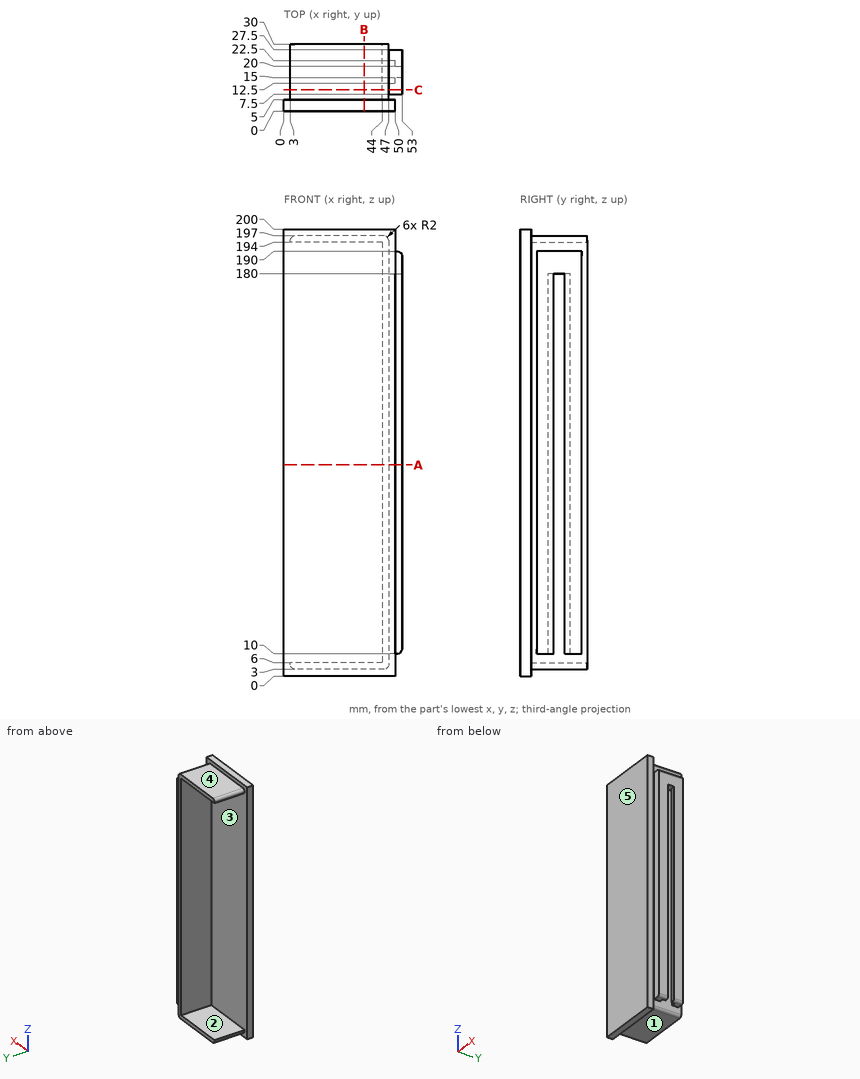
Here's the drawing with two shaded views (mm, measured from the low corner). I have some questions. A direction names the side the tool comes from. Give positions to 0.01 mm unless a question says otherwise; leave off trailing zeros. Write each loop counter-clockwise with the first axis right and the second up, starting at its lowest first coordinate (ties: lowest second). Pieces come first, ordered by that corner, then holes. Notation, with made-up numbers: (-30, 14.25) -> (0, 14.25) arc R25 cw to (0, 37.25) -> close; hole circle Ø5 at (89, -29). An arc over 180 degrees is marked (long way). Use one line per item in the form item = value.
1) Suppose I cut it at A-A (z = 94.5). Please give me the cut outline in (x, y).
Verdict:
outline = (0, 0) -> (50, 0) -> (50, 5) -> (47, 5) -> (47, 7.5) -> (53, 7.5) -> (53, 15) -> (50, 15) -> (50, 12.5) -> (47, 12.5) -> (47, 22.5) -> (50, 22.5) -> (50, 20) -> (53, 20) -> (53, 27.5) -> (47, 27.5) -> (47, 30) -> (44, 30) -> (44, 5) -> (0, 5) -> close
2) If I drill on L1, parallel to Z at x = 15, y = 18.75; L2, parallel to X at y = 14.5, z = 120.5; L3, parallel to Y at x = 10, z = 70, over which ranges is the centre line in solid material (lowest first)? Write a range as [from, to].
Verdict:
L1 = [3, 6], [194, 197]
L2 = [44, 47], [50, 53]
L3 = [0, 5]
3) Suppose I cut it at B-B (x = 36). Please give me the cut outline in (y, z), and give its area (3 significant figures).
Verdict:
outline = (0, 0) -> (5, 0) -> (5, 3) -> (30, 3) -> (30, 6) -> (5, 6) -> (5, 194) -> (30, 194) -> (30, 197) -> (5, 197) -> (5, 200) -> (0, 200) -> close
area = 1,150 mm2
4) We'd pull the mould along Z, two halves only. Please class the marked faces 3, 4 and 5: +Z half, -Z half, draft (parallel to the pull), parting line (faces both ways), or undercut.
Verdict:
face_3 = undercut
face_4 = +Z half
face_5 = draft
5) I'm going to push flat-ended pins straight in: pin 1 (4 mm diameter, centred on y = 2, z = 85, fed in from +X); pin 2 (5 mm diameter, centred on x = 23.5, z = 117.5, fed in from +Y); pin 3 (0.8 mm diameter, centred on y = 17.5, z = 5.5, fed in from -X). Where does each tip first touch, or does it pass through?
Verdict:
pin_1 = 50
pin_2 = 5
pin_3 = 3
6) Suppose I cut it at C-C (y = 9.5). Please give me the cut outline in (x, z).
Verdict:
outline = (3, 5) arc R2 ccw to (5, 3) -> (45, 3) arc R2 ccw to (47, 5) -> (47, 10) -> (51, 10) arc R2 ccw to (53, 12) -> (53, 188) arc R2 ccw to (51, 190) -> (47, 190) -> (47, 195) arc R2 ccw to (45, 197) -> (5, 197) arc R2 ccw to (3, 195) -> (3, 194) -> (44, 194) -> (44, 6) -> (3, 6) -> close
7) On a 3-axis mill with a long thin cutter (end or side, diameter ignored), from which of +Z, -Z, +X, -X, +Y, -Y can I reach the whole of each face in a straight line? I mean the marked faces 1 and 2. Say none if no direction works.
Verdict:
face_1 = -Z, +X, -X, +Y
face_2 = -X, +Y
